```python
from build123d import *

# Parameters (mm, degrees)
EXTRUDE_1_DEPTH     = 6
CUT_EXTRUDE_1_DEPTH = 248.560093715
SKETCH_3_W          = 6
SKETCH_3_H          = 120
EXTRUDE_2_DEPTH     = 21
SKETCH_4_W          = 120
SKETCH_4_H          = 6
EXTRUDE_3_DEPTH     = 21
SKETCH_5_R          = 1.6
CUT_EXTRUDE_2_DEPTH = 248.560093715
SKETCH_6_R          = 3
CUT_EXTRUDE_3_DEPTH = 3


with BuildPart() as part:
    # 草圖1 → 填料-伸長1 (new body)
    with BuildSketch(Plane.XY):
        with BuildLine():
            Line((0, 0), (0, -175))
            ThreePointArc((0, -175), (151.554445662, -87.5), (151.554445662, 87.5))
            Line((151.554445662, 87.5), (0, 0))
        make_face()
    extrude(amount=EXTRUDE_1_DEPTH)

    # 草圖2 → 除料-伸長1 (cut, through all)
    with BuildSketch(Plane.XY.offset(6)):
        with BuildLine():
            Line((0, 0), (0, -55))
            ThreePointArc((0, -55), (27.500000113, -47.631397143), (47.631397339, -27.499999773))
            ThreePointArc((47.631397339, -27.499999773), (53.12592048, -14.235047354), (55, 0))
            ThreePointArc((55, 0), (53.125920434, 14.235047524), (47.631397163, 27.500000078))
            Line((47.631397208, 27.5), (0, 0))
        make_face()
        with BuildLine():
            ThreePointArc((0, 55), (-55, 0), (0, -55))
            Line((0, -55), (0, 0))
            Line((0, 0), (47.631397208, 27.5))
            ThreePointArc((47.631397163, 27.500000078), (27.499999961, 47.631397231), (0, 55))
        make_face()
        with BuildLine():
            ThreePointArc((47.631397339, -27.499999773), (27.500000113, -47.631397143), (0, -55))
            Line((0, -55), (31.754264805, -55))
            Line((31.754264805, -55), (47.631397339, -27.499999773))
        make_face()
        with BuildLine():
            ThreePointArc((55, 0), (53.12592048, -14.235047354), (47.631397339, -27.499999773))
            Line((47.631397339, -27.499999773), (63.508529611, 0))
            Line((63.508529611, 0), (47.631397163, 27.500000078))
            ThreePointArc((47.631397163, 27.500000078), (53.125920434, 14.235047524), (55, 0))
        make_face()
    extrude(amount=-CUT_EXTRUDE_1_DEPTH, mode=Mode.SUBTRACT)

    # 草圖3 → 填料-伸長2 (add)
    with BuildSketch(Plane.ZY):
        with Locations((3, -115)):
            Rectangle(SKETCH_3_W, SKETCH_3_H)
    extrude(amount=EXTRUDE_2_DEPTH)

    # 草圖4 → 填料-伸長3 (add)
    with BuildSketch(Plane(origin=(0, 0, 0), x_dir=(0.8660254037844362, 0.5000000000000046, 0), z_dir=(-0.5000000000000044, 0.866025403784436, 0))):
        with Locations((115, -3)):
            Rectangle(SKETCH_4_W, SKETCH_4_H)
    extrude(amount=EXTRUDE_3_DEPTH)

    # 草圖5 → 除料-伸長2 (cut, through all)
    with BuildSketch(Plane.XY.offset(6)):
        with Locations((61.229349178, -147.820725202)):
            Circle(SKETCH_5_R)
        with Locations((26.787840266, -64.671567276)):
            Circle(SKETCH_5_R)
        with Locations(Location((158.63117782, 20.884190755, 0), (0, 0, 180))):
            Circle(SKETCH_5_R)
        with Locations(Location((69.401140296, 9.136833455, 0), (0, 0, 180))):
            Circle(SKETCH_5_R)
    extrude(amount=-CUT_EXTRUDE_2_DEPTH, mode=Mode.SUBTRACT)

    # 草圖6 → 除料-伸長3 (cut)
    with BuildSketch(Plane.XY.offset(6)):
        with Locations((61.229349178, -147.820725202)):
            Circle(SKETCH_6_R)
        with Locations((26.787840266, -64.671567276)):
            Circle(SKETCH_6_R)
        with Locations((69.401140296, 9.136833455)):
            Circle(SKETCH_6_R)
        with Locations((158.63117782, 20.884190755)):
            Circle(SKETCH_6_R)
    extrude(amount=-CUT_EXTRUDE_3_DEPTH, mode=Mode.SUBTRACT)


solid = part.part
```
Input: part model. Units: mm. Frame: model coordinates. A direction names the side the tool comes from. Coordinates: 2 decimals unless noted, no trailing zeros. Write each loop counter-clockwise with the first axis right and the second up, starting at its lowest first coordinate (ties: lowest second). Pieces come first, ordered by that corner, then holes. Notation, with made-up numbers: (23, 18.25) -> (47, 18.25) arc R17 ccw to (47, 46.25) -> close; hole circle Ø8 at (-38, 36.25). An arc over 180 degrees is marked (long way). Answer as a JSON object with one key per item and string values.
1. Section D-D on x = 123. Return the cut outline in (y, z).
Result set:
{"outline": "(-124.48, 0) -> (95.26, 0) -> (95.26, 6) -> (-124.48, 6) -> close"}
2. Section B-B on z = 4.5. Return the cut outline in (x, y).
Result set:
{"outline": "(-21, -175) -> (0, -175) arc R175 ccw to (151.55, 87.5) -> (141.05, 105.69) -> (37.13, 45.69) -> (63.51, 0) -> (31.75, -55) -> (-21, -55) -> close; hole circle Ø6 at (26.79, -64.67); hole circle Ø6 at (61.23, -147.82); hole circle Ø6 at (69.4, 9.14); hole circle Ø6 at (158.63, 20.88)"}
3. First-contact query: P1, Ø1.8, axis at x = 69.5, y = 10, coming from the +Z side; P2, Ø1.8, axis at x = 7, z = 2, coming from the +Y side; P3, Ø2, axis at x = 59, z = 0.5, coming from the -Y side. Flat tips, straight axial feed; report the tip coordinate or a pass-through.
Result set:
{"P1": "stops at z = 3", "P2": "stops at y = -55", "P3": "stops at y = -165.11"}
4. Access query for faces 1 (the face through (28, -66, 3)), 2 (the face through (146.378, 96.466, 3.042)), 3 (the face through (6, -55, 3)). Directions: +Z, -Z, +X, -X, +Y, -Y. A direction counts if a zero-diameter tool reaches every point of the face in a straight line with its end or side. Return the directions, or none.
Result set:
{"face 1": "+Z", "face 2": "+Z, -Z, +X, +Y", "face 3": "+Z, -Z, -X, +Y"}
5. Section A-A on x = 44. Return the cut outline in (y, z).
Result set:
{"outline": "(-169.38, 0) -> (-33.79, 0) -> (-33.79, 6) -> (-169.38, 6) -> close; (33.79, 0) -> (49.65, 0) -> (49.65, 6) -> (33.79, 6) -> close"}
6. Section C-C on y = -126. Return the cut outline in (x, z).
Result set:
{"outline": "(-21, 0) -> (121.45, 0) -> (121.45, 6) -> (-21, 6) -> close"}
7. Material intervals for line 1 (Y direction, x = 71, z = 4); line 2 (Y direction, x = 51, z = 3.75); line 3 (X direction, y = -3, z = 2), sorted ascending. Write a range as from..to.
Result set:
{"line 1": "y = -159.95..6.6, 11.68..65.24", "line 2": "y = -167.4..-21.67, 21.67..53.69", "line 3": "x = 61.78..174.97"}
8. Mould query, pull axis X, two halves, no side actions, for faces 4 (the face through (150.255, -89.712, 2.958)), 5 (the face through (72.26, 10.04, 4.52)), 6 (the face through (28.4, -62.14, 4.52)), 7 (the face through (88.37, 75.27, 2.96)). Classes: released by +X, released by -X, zero draft, split by the parting line, or undercut.
Result set:
{"face 4": "released by +X", "face 5": "undercut", "face 6": "undercut", "face 7": "released by -X"}
